```python
from build123d import *

# Parameters (mm, degrees)
SKETCH1_R           = 2.35
BOSS_EXTRUDE1_DEPTH = 7.8
SKETCH2_R           = 2.705
CUT_EXTRUDE2_DEPTH  = 0.7
CUT_EXTRUDE3_START  = -0.7
SKETCH3_R           = 2.705
CUT_EXTRUDE3_DEPTH  = 0.7


with BuildPart() as part:
    # Sketch1 → Boss-Extrude1 (new body)
    with BuildSketch(Plane(origin=(0, 0, 0), x_dir=(0, 0, -1), z_dir=(1, 0, 0))):
        with BuildLine():
            Line((-24, -3.73), (24, -3.73))
            ThreePointArc((24, -3.73), (27.73, 0), (24, 3.73))
            Line((24, 3.73), (-24, 3.73))
            ThreePointArc((-24, 3.73), (-27.73, 0), (-24, -3.73))
        make_face()
        with Locations((-24, 0)):
            Circle(SKETCH1_R, mode=Mode.SUBTRACT)
        with Locations((-16, 0)):
            Circle(SKETCH1_R, mode=Mode.SUBTRACT)
        with Locations((-8, 0)):
            Circle(SKETCH1_R, mode=Mode.SUBTRACT)
        Circle(SKETCH1_R, mode=Mode.SUBTRACT)
        with Locations((8, 0)):
            Circle(SKETCH1_R, mode=Mode.SUBTRACT)
        with Locations((16, 0)):
            Circle(SKETCH1_R, mode=Mode.SUBTRACT)
        with Locations((24, 0)):
            Circle(SKETCH1_R, mode=Mode.SUBTRACT)
    extrude(amount=BOSS_EXTRUDE1_DEPTH)

    # Sketch2 → Cut-Extrude2 (cut)
    with BuildSketch(Plane.ZY):
        with Locations((-24, 0)):
            Circle(SKETCH2_R)
        with Locations((-16, 0)):
            Circle(SKETCH2_R)
        with Locations((-8, 0)):
            Circle(SKETCH2_R)
        Circle(SKETCH2_R)
        with Locations((8, 0)):
            Circle(SKETCH2_R)
        with Locations((16, 0)):
            Circle(SKETCH2_R)
        with Locations((24, 0)):
            Circle(SKETCH2_R)
    extrude(amount=-CUT_EXTRUDE2_DEPTH, mode=Mode.SUBTRACT)

    # Sketch3 → Cut-Extrude3 (cut)
    with BuildSketch(Plane(origin=(7.8, 0, 0), x_dir=(0, 0, -1), z_dir=(1, 0, 0)).offset(CUT_EXTRUDE3_START)):
        with Locations(Location((-24, 0, 0), (0, 0, 180))):
            Circle(SKETCH3_R)
        with Locations(Location((-16, 0, 0), (0, 0, 180))):
            Circle(SKETCH3_R)
        with Locations(Location((-8, 0, 0), (0, 0, 180))):
            Circle(SKETCH3_R)
        with Locations(Location((0, 0, 0), (0, 0, 180))):
            Circle(SKETCH3_R)
        with Locations(Location((8, 0, 0), (0, 0, 180))):
            Circle(SKETCH3_R)
        with Locations(Location((16, 0, 0), (0, 0, 180))):
            Circle(SKETCH3_R)
        with Locations(Location((24, 0, 0), (0, 0, 180))):
            Circle(SKETCH3_R)
    extrude(amount=CUT_EXTRUDE3_DEPTH, mode=Mode.SUBTRACT)


solid = part.part
```
Design review of the part built by this model. Coordinates are the model's own, in mm. A direction names the side the tool comes from. Give positions to 0.01 mm unless a question says otherwise; leave off trailing zeros. Order: outer loops, then holes, each group sorted by start corner. A loop starts at its lowest first (then second) coordinate and runs counter-clockwise, first axis right, second up. Notation, with made-up numbers: (73, 51.5) - (127, 51.5) arc R8 ccw to (127, 57.5) - close; hole circle Ø8 at (-15, 33.25). An arc over 180 degrees is marked (long way). Use a Markdown table: item, result. Add a question column.
(1) Wall thickness on probe 1 along Y at (x, z) = (5.5, 16); probe 2 along Y at (x, z) = (7.6, -24) (3 decimals); probe 3 along X at (y, z) = (1.75, 22): over which ranges is each line inside the solid? List them lowest first. Write a range as [from, to].
(2) Add section B-B on x = 3.75. Give the boundary of the cut face in (y, z), then the cut area to 3 significant figures.
(3) Add section A-A on z = -16. Give the boundary of the cut face in (x, y) (3 decimals), then the cut area to 3 significant figures.
(4) Add section D-D on z = 9. Give the boundary of the cut face in (x, y).
(5) Add section C-C on y = -1.75. Give the number of separate pieces and of enclosed holes in the cut face, then the cut area to 3 significant figures.
(6) Machinability: for faces 1 (the face through (3.855, 0.103, -21.652)), 2 (the face through (7.445, -0.119, -26.702)), 3 (the face through (0.345, 0.119, -26.702)), which of the approach directions +Z, -Z, +X, -X, +Y, -Y give a long, thin tool a straight path to every point of the face, cutting with its end or side? Answer none if there is none.
(7) Mouldability with a two-part tool opening along Z and no side actions: class faces 4 (the face through (4, -3.73, 0)), 5 (the face through (3.85, -0.08, -27.73)), 6 (the face through (7.45, -0.81, 10.58)), 7 (the face through (3.85, 0.08, 27.73)) as +Z half, -Z half, draft (parallel to the pull), parting line (faces both ways), or undercut.
Report:
| question | item | result |
|---|---|---|
| 1 | probe 1 | y = [-3.73, -2.35], [2.35, 3.73] |
| 1 | probe 2 | y = [-3.73, -2.705], [2.705, 3.73] |
| 1 | probe 3 | x = [0.7, 7.1] |
| 2 | outline | (-3.73, -24) arc R3.73 ccw to (3.73, -24) - (3.73, 24) arc R3.73 ccw to (-3.73, 24) - close; hole circle Ø4.7 at (0, -24); hole circle Ø4.7 at (0, -16); hole circle Ø4.7 at (0, -8); hole circle Ø4.7 at (0, 0); hole circle Ø4.7 at (0, 8); hole circle Ø4.7 at (0, 16); hole circle Ø4.7 at (0, 24) |
| 2 | area | 280 mm² |
| 3 | outline | (0, -3.73) - (7.8, -3.73) - (7.8, -2.705) - (7.1, -2.705) - (7.1, -2.35) - (0.7, -2.35) - (0.7, -2.705) - (0, -2.705) - close; (0, 2.705) - (0.7, 2.705) - (0.7, 2.35) - (7.1, 2.35) - (7.1, 2.705) - (7.8, 2.705) - (7.8, 3.73) - (0, 3.73) - close |
| 3 | area | 20.5 mm² |
| 4 | outline | (0, -3.73) - (7.8, -3.73) - (7.8, -2.51) - (7.1, -2.51) - (7.1, -2.13) - (0.7, -2.13) - (0.7, -2.51) - (0, -2.51) - close; (0, 2.51) - (0.7, 2.51) - (0.7, 2.13) - (7.1, 2.13) - (7.1, 2.51) - (7.8, 2.51) - (7.8, 3.73) - (0, 3.73) - close |
| 5 | separate pieces | 8 |
| 5 | enclosed holes | 0 |
| 5 | area | 245 mm² |
| 6 | face 1 | +X, -X |
| 6 | face 2 | +X |
| 6 | face 3 | -X |
| 7 | face 4 | draft |
| 7 | face 5 | -Z half |
| 7 | face 6 | undercut |
| 7 | face 7 | +Z half |
